Read the model definition and answer for the solid it produces. Units are mm, in the model's axes. A direction names the side the tool comes from. Coordinates: 2 decimals unless noted, no trailing zeros. Write each loop counter-clockwise with the first axis right and the second up, starting at its lowest first coordinate (ties: lowest second). Pieces come first, ordered by that corner, then holes.
from build123d import *

# Parameters (mm, degrees)
SKETCH1_W           = 1.5
SKETCH1_H           = 70
BOSS_EXTRUDE1_DEPTH = 5
SKETCH1_3_W         = 101.5
SKETCH1_3_H         = 70
BOSS_EXTRUDE2_DEPTH = 1.5
BOSS_EXTRUDE3_START = 1.5
SKETCH1_4_W         = 1.5
SKETCH1_4_H         = 70
BOSS_EXTRUDE3_DEPTH = 10
SKETCH2_W           = 10
SKETCH2_H           = 5
BOSS_EXTRUDE4_DEPTH = 1.5
BOSS_EXTRUDE5_START = -1.5
SKETCH2_4_W         = 10
SKETCH2_4_H         = 5
BOSS_EXTRUDE5_DEPTH = 3.5
SKETCH4_R           = 4.95
SKETCH4_R_2         = 2.5
CUT_EXTRUDE1_DEPTH  = 1.5
SKETCH4_2_R         = 2.5
CUT_EXTRUDE2_DEPTH  = 106.785569976


with BuildPart() as part:
    # Sketch1 → Boss-Extrude1 (new body)
    with BuildSketch(Plane(origin=(0, 0, 0), x_dir=(1, 0, 0), z_dir=(0, 1, 0))):
        with Locations((-63.901879758, 5.076012966)):
            Rectangle(SKETCH1_W, SKETCH1_H)
    extrude(amount=-BOSS_EXTRUDE1_DEPTH)

    # Sketch1<3> → Boss-Extrude2 (add)
    with BuildSketch(Plane(origin=(0, 0, 0), x_dir=(1, 0, 0), z_dir=(0, 1, 0))):
        with Locations((-13.901879758, 5.076012966)):
            Rectangle(SKETCH1_3_W, SKETCH1_3_H)
    extrude(amount=BOSS_EXTRUDE2_DEPTH)

    # Sketch1<4> → Boss-Extrude3 (add)
    with BuildSketch(Plane(origin=(0, 0, 0), x_dir=(1, 0, 0), z_dir=(0, 1, 0)).offset(BOSS_EXTRUDE3_START)):
        with Locations((36.098120242, 5.076012966)):
            Rectangle(SKETCH1_4_W, SKETCH1_4_H)
    extrude(amount=BOSS_EXTRUDE3_DEPTH)

    # Sketch2 → Boss-Extrude4 (add)
    with BuildSketch(Plane(origin=(36.848120242, 0, 0), x_dir=(0, 0, -1), z_dir=(1, 0, 0))):
        with Locations((-9.923987034, 14)):
            Rectangle(SKETCH2_W, SKETCH2_H)
        with Locations((20.076012966, 14)):
            Rectangle(SKETCH2_W, SKETCH2_H)
    extrude(amount=-BOSS_EXTRUDE4_DEPTH)

    # Sketch2<4> → Boss-Extrude5 (add)
    with BuildSketch(Plane(origin=(36.848120242, 0, 0), x_dir=(0, 0, -1), z_dir=(1, 0, 0)).offset(BOSS_EXTRUDE5_START)):
        with Locations((-9.923987034, 14)):
            Rectangle(SKETCH2_4_W, SKETCH2_4_H)
        with Locations((-9.923987034, 9)):
            Rectangle(SKETCH2_4_W, SKETCH2_4_H)
        with Locations((20.076012966, 9)):
            Rectangle(SKETCH2_4_W, SKETCH2_4_H)
        with Locations((20.076012966, 14)):
            Rectangle(SKETCH2_4_W, SKETCH2_4_H)
        with Locations((-9.923987034, 4)):
            Rectangle(SKETCH2_4_W, SKETCH2_4_H)
        with Locations((20.076012966, 4)):
            Rectangle(SKETCH2_4_W, SKETCH2_4_H)
    extrude(amount=-BOSS_EXTRUDE5_DEPTH)

    # Sketch4 → Cut-Extrude1 (cut)
    # profile 1 of 2: a face of its own
    with BuildSketch(Plane.ZY.offset(-31.848120242)):
        with Locations((-20.076012966, 11.5)):
            Circle(SKETCH4_R)
        with Locations((-20.076012966, 11.5)):
            Circle(SKETCH4_R_2, mode=Mode.SUBTRACT)
    # profile 2 of 2: a face of its own
    with BuildSketch(Plane.ZY.offset(-31.848120242)):
        with Locations((9.923987034, 11.5)):
            Circle(SKETCH4_R)
        with Locations((9.923987034, 11.5)):
            Circle(SKETCH4_R_2, mode=Mode.SUBTRACT)
    extrude(amount=-CUT_EXTRUDE1_DEPTH, mode=Mode.SUBTRACT)

    # Sketch4<2> → Cut-Extrude2 (cut, through all)
    with BuildSketch(Plane.ZY.offset(-31.848120242)):
        with Locations((-20.076012966, 11.5)):
            Circle(SKETCH4_2_R)
        with Locations((9.923987034, 11.5)):
            Circle(SKETCH4_2_R)
    extrude(amount=-CUT_EXTRUDE2_DEPTH, mode=Mode.SUBTRACT)


solid = part.part
Item 1: Given pin 1 (8 mm diameter, centred on y = 14, z = 12, fed in from -X); pin 2 (2.5 mm diameter, centred on x = 34, y = 10, fed in from +Z); pin 3 (5 mm diameter, centred on y = 5, z = -31, fed in from -X); pin 4 (4 mm diameter, centred on y = 11.5, z = 9.92, fed in from -X), each flat-ended and moving along its own axis, determine where each tip first touches the part or whether it passes through.
Item 2: For faces 5 (the flat face through (33.348, 14, 9)), 6 (the flat face through (34, 9, 4.924)), 7 (the flat face through (31.848, 6, 10)), 8 (the flat face through (35.348, 6, 23)), 9 (the flat face through (-63.152, -2, -5)), determine the directions among +Z, -Z, +X, -X, +Y, -Y from which every point of the face is accessible in a straight line to the end or side of a thin tool.
Item 3: Find the intervals of material crossed by probe 1 along X at (y, z) = (-3.75, -22); probe 2 along X at (y, z) = (2.5, 20.5); probe 3 along Y at (x, z) = (-41, -3), in increasing order.
Item 4: The part is cut by section A-A (z = -6.5). Give the vertices of the cut face in (x, y), and give its area (3 significant figures).
Item 5: Determine the mould class of faces 1 (the flat face through (35.348, 6, -32)), 2 (the flat face through (-14, 0, -6)), 3 (the cylindrical face through (35.07, 9.98, -22.06)), 4 (the flat face through (33.348, 14, -21)) for opening direction Y: +Y half, -Y half, draft (parallel to the pull), parting line (faces both ways), or undercut.
Item 6: The part is cut by section B-B (x = 0.5). Give the vertices of the cut face in (y, z), and give its area (3 significant figures).
Answer:
1. pin 1: stops at x = 31.85
1. pin 2: stops at z = 14.92
1. pin 3: stops at x = 35.35
1. pin 4: passes through
2. face 5: -X
2. face 6: -X, +Y
2. face 7: +Z, -Z, -X, +Y
2. face 8: +Z, -X, +Y
2. face 9: +Z, -Z, +X, -Y
3. probe 1: x = -64.65 to -63.15
3. probe 2: x = 35.35 to 36.85
3. probe 3: y = 0 to 1.5
4. outline: (-64.65, -5) - (-63.15, -5) - (-63.15, 0) - (36.85, 0) - (36.85, 11.5) - (35.35, 11.5) - (35.35, 1.5) - (-64.65, 1.5) - close
4. area: 175 mm2
5. face 1: draft
5. face 2: -Y half
5. face 3: undercut
5. face 4: undercut
6. outline: (0, -40.08) - (1.5, -40.08) - (1.5, 29.92) - (0, 29.92) - close
6. area: 105 mm2
